```python
from build123d import *

# Parameters (mm, degrees)
SKETCH1_W                                = 178
SKETCH1_H                                = 76
BOSS_EXTRUDE1_DEPTH                      = 90
BOSS_EXTRUDE2_DEPTH                      = 14
CBORE_FOR_M14_HEX_HEAD_BOLT1_D           = 16
CBORE_FOR_M14_HEX_HEAD_BOLT1_CBORE_D     = 28
CBORE_FOR_M14_HEX_HEAD_BOLT1_CBORE_DEPTH = 2
SKETCH4_W                                = 160
SKETCH4_H                                = 60
CUT_EXTRUDE1_DEPTH                       = 63
SKETCH5_W                                = 180
SKETCH5_H                                = 86
SKETCH5_W_2                              = 178
SKETCH5_H_2                              = 76
BOSS_EXTRUDE4_DEPTH                      = 12


with BuildPart() as part:
    # Sketch1 → Boss-Extrude1 (new body)
    with BuildSketch(Plane(origin=(0, 0, 0), x_dir=(1, 0, 0), z_dir=(0, 1, 0))):
        Rectangle(SKETCH1_W, SKETCH1_H)
    extrude(amount=BOSS_EXTRUDE1_DEPTH)

    # Sketch2 → Boss-Extrude2 (add)
    with BuildSketch(Plane(origin=(0, 0, 0), x_dir=(1, 0, 0), z_dir=(0, 1, 0))):
        with BuildLine():
            Line((123.89505406, 15.036219776), (89, 38))
            Line((89, 38), (89, -38))
            Line((89, -38), (123.89505406, -15.036219776))
            ThreePointArc((123.89505406, -15.036219776), (132, 0), (123.89505406, 15.036219776))
        make_face()
    boss_extrude2 = extrude(amount=BOSS_EXTRUDE2_DEPTH)

    # CBORE for M14 Hex Head Bolt1 (through all)
    with Locations(Plane(origin=(114, 14, 0), x_dir=(0, 0, 1), z_dir=(0, 1, 0))):
        with Locations((0, 0)):
            cbore_for_m14_hex_head_bolt1 = CounterBoreHole(CBORE_FOR_M14_HEX_HEAD_BOLT1_D / 2, CBORE_FOR_M14_HEX_HEAD_BOLT1_CBORE_D / 2, CBORE_FOR_M14_HEX_HEAD_BOLT1_CBORE_DEPTH)

    # Mirror1: Boss-Extrude2, CBORE for M14 Hex Head Bolt1 across plane
    add(boss_extrude2.mirror(Plane(origin=(0, 0, 0), x_dir=(0, 0, 1), z_dir=(1, 0, 0))))
    add(cbore_for_m14_hex_head_bolt1.mirror(Plane(origin=(0, 0, 0), x_dir=(0, 0, 1), z_dir=(1, 0, 0))), mode=Mode.SUBTRACT)

    # Sketch4 → Cut-Extrude1 (cut)
    with BuildSketch(Plane(origin=(0, 90, 0), x_dir=(1, 0, 0), z_dir=(0, 1, 0))):
        Rectangle(SKETCH4_W, SKETCH4_H)
    extrude(amount=-CUT_EXTRUDE1_DEPTH, mode=Mode.SUBTRACT)

    # Sketch5 → Boss-Extrude4 (add)
    # profile 1 of 6: a face of its own
    with BuildSketch(Plane(origin=(0, 90, 0), x_dir=(1, 0, 0), z_dir=(0, 1, 0))):
        Rectangle(SKETCH5_W, SKETCH5_H)
        Rectangle(SKETCH5_W_2, SKETCH5_H_2, mode=Mode.SUBTRACT)
    # profile 2 of 6: a face of its own
    with BuildSketch(Plane(origin=(0, 90, 0), x_dir=(1, 0, 0), z_dir=(0, 1, 0))):
        Rectangle(SKETCH5_W_2, SKETCH5_H_2)
        Polygon((70, -30), (-70, -30), (-80, -30), (-80, -20), (-80, 20), (-80, 30), (-70, 30), (70, 30), (80, 30), (80, 20), (80, -20), (80, -30), align=None, mode=Mode.SUBTRACT)
    # profile 3 of 6: a face of its own
    with BuildSketch(Plane(origin=(0, 90, 0), x_dir=(1, 0, 0), z_dir=(0, 1, 0))):
        with BuildLine():
            Line((-80, 30), (-80, 20))
            ThreePointArc((-80, 20), (-72.928932188, 22.928932188), (-70, 30))
            Line((-70, 30), (-80, 30))
        make_face()
    # profile 4 of 6: a face of its own
    with BuildSketch(Plane(origin=(0, 90, 0), x_dir=(1, 0, 0), z_dir=(0, 1, 0))):
        with BuildLine():
            Line((-80, -30), (-70, -30))
            ThreePointArc((-70, -30), (-72.928932188, -22.928932188), (-80, -20))
            Line((-80, -20), (-80, -30))
        make_face()
    # profile 5 of 6: a face of its own
    with BuildSketch(Plane(origin=(0, 90, 0), x_dir=(1, 0, 0), z_dir=(0, 1, 0))):
        with BuildLine():
            ThreePointArc((80, -20), (72.928932188, -22.928932188), (70, -30))
            Line((70, -30), (80, -30))
            Line((80, -30), (80, -20))
        make_face()
    # profile 6 of 6: a face of its own
    with BuildSketch(Plane(origin=(0, 90, 0), x_dir=(1, 0, 0), z_dir=(0, 1, 0))):
        with BuildLine():
            ThreePointArc((70, 30), (72.928932188, 22.928932188), (80, 20))
            Line((80, 20), (80, 30))
            Line((80, 30), (70, 30))
        make_face()
    extrude(amount=BOSS_EXTRUDE4_DEPTH)


solid = part.part
```
The listing builds one solid part. Answer for the finished solid, in the listing's coordinates (mm). A direction names the side the tool comes from. Coordinates: 2 decimals unless noted, no trailing zeros. Loops run counter-clockwise (first coordinate to the right, second up) from the corner with the lowest first, then second, coordinate; pieces in that order, holes last. Notation, with made-up numbers: (45.5, 24.25) - (86.5, 24.25) arc R32 ccw to (86.5, 53.25) - close; hole circle Ø2 at (77.5, 0.5). An arc over 180 degrees is marked (long way). Use a Markdown table: item, result. Add a question column.
1) The part is cut by section B-B, the plane z = 3. State how many separate pieces and enclosed holes the cut face has, and give its area (3 significant figures).
2) The part is cut by section A-A, the plane y = 82.5. Give the vertices of the cut face in (x, z), and give its area (3 significant figures).
3) Given pin 1 (4 mm diameter, centred on x = -9.5, z = 10.5, fed in from +Y); pin 2 (1 mm diameter, centred on y = 40.5, z = 29.5, fed in from +X); pin 3 (5 mm diameter, centred on x = 73, z = 25, fed in from -Y); pin 4 (4 mm diameter, centred on x = 90.5, y = 80, fed in from +Z), each flat-ended and moving along its own axis, determine where each tip first touches the part or whether it passes through.
4) The part is cut by section C-C, the plane x = -62.5. Give the vertices of the cut face in (y, z), and give its area (3 significant figures).
5) The mould has two halves that part along Y. Classify faces 6 (the flat face through (-80, 64, 0)), 7 (the flat face through (76, 90, 26)), 8 (the cylindrical face through (-73.01, 95.92, -22.85)), 9 (the flat face through (-108, 12, 6)): released by +Y, released by -Y, zero draft, split by the parting line, or undercut.
6) For faces 1 (the cylindrical face through (-132, 7, 0)), 2 (the flat face through (-90, 96, 1)), 3 (the flat face through (-1, 96, 43)), 4 (the flat face through (-89, 51, 1)), 5 (the cylindrical face through (73.01, 95.92, 22.85)), determine the directions among +Z, -Z, +X, -X, +Y, -Y from which every point of the face is accessible in a straight line to the end or side of a thin tool.
7) Find the intervals of material crossed by line 1 (X direction, y = 92.5, z = -8); line 2 (X direction, y = 78, z = 7.5); line 3 (Z direction, x = 68, y = 63.5), in increasing order.
8) The part is cut by section D-D, the plane x = -114. Give the vertices of the cut face in (y, z).
Here are the results:
| question | item | result |
|---|---|---|
| 1 | separate pieces | 3 |
| 1 | enclosed holes | 0 |
| 1 | area | 6,910 mm^2 |
| 2 | outline | (-89, -38) - (89, -38) - (89, 38) - (-89, 38) - close; hole (-80, -30) - (80, -30) - (80, 30) - (-80, 30) - close |
| 2 | area | 3,930 mm^2 |
| 3 | pin 1 | stops at y = 27 |
| 3 | pin 2 | stops at x = 89 |
| 3 | pin 3 | stops at y = 0 |
| 3 | pin 4 | stops at z = 38 |
| 4 | outline | (0, -38) - (90, -38) - (90, -43) - (102, -43) - (102, -30) - (27, -30) - (27, 30) - (102, 30) - (102, 43) - (90, 43) - (90, 38) - (0, 38) - close |
| 4 | area | 3,370 mm^2 |
| 5 | face 6 | undercut |
| 5 | face 7 | undercut |
| 5 | face 8 | zero draft |
| 5 | face 9 | released by +Y |
| 6 | face 1 | -X, +Y, -Y |
| 6 | face 2 | +Z, -Z, -X, +Y |
| 6 | face 3 | +Z, +X, -X, +Y, -Y |
| 6 | face 4 | +Z, -Z, -X |
| 6 | face 5 | +Y |
| 7 | line 1 | x = -90 to -80, 80 to 90 |
| 7 | line 2 | x = -89 to -80, 80 to 89 |
| 7 | line 3 | z = -38 to -30, 30 to 38 |
| 8 | outline | (0, -21.55) - (14, -21.55) - (14, -14) - (12, -14) - (12, -8) - (0, -8) - close; (0, 8) - (12, 8) - (12, 14) - (14, 14) - (14, 21.55) - (0, 21.55) - close |
